Build history of the part. All positions in model axes, mm. Face numbers are marked on the shaded views. Coordinates: 2 decimals unless noted, no trailing zeros. Loops run counter-clockwise (first coordinate to the right, second up) from the corner with the lowest first, then second, coordinate; pieces in that order, holes last.
(1) Slice it at C-C (z = 15). Give the cut face in (x, y).
(2) Slice it at D-D (z = 11). Give the cut face in (x, y), and give its area (3 significant figures).
(3) Slice it at A-A (x = 0). Give the cut face in (y, z), and give its area (3 significant figures).
(4) Flat gauge pins, fed straight in: P1, Ø11, axis at x = 0, y = -14.82, coming from the +Z side; P2, Ø1, axis at y = -45.5, z = 16, coming from the -X side; P3, Ø5, axis at y = -46.5, z = -7, coming from the +X side. Where does each tip first touch, or does it go through?
(5) Wall check: L1, parallel to Y at x = 0, z = 14.25; L2, parallel to Y at x = -5.5, z = 10.5; L3, parallel to X at y = -37, z = 17. Give the ranges that are in metal, low to high.
(6) Two-plate mould, pull along Y, no slides. Class the marked faces 1, 2 and 3: pulls with the +Y half, pulls with the -Y half, needs draft (parallel to the pull), parting line crosses it, or undercut.
(7) Slice it at B-B (y = -44). Give the cut face in (x, z), and give its area (3 significant figures).
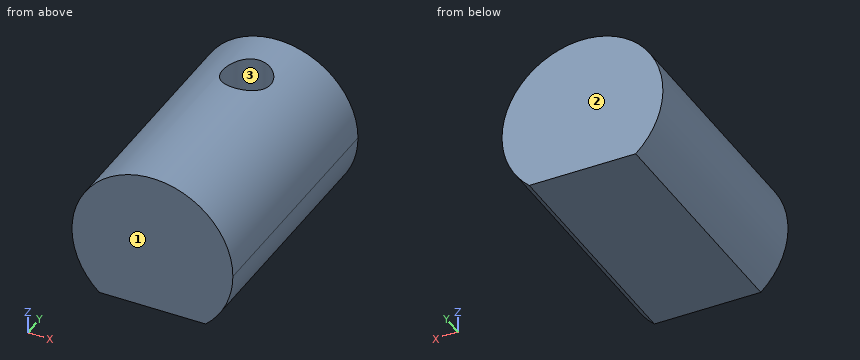
from build123d import *

# Parameters (mm, degrees)
F0_R     = 20
F1_DEPTH = 60
F3_R     = 6
F4_DEPTH = 23.59607
F5_W     = 79.34783
F5_H     = 17.173914
F6_DEPTH = 121.24079


with BuildPart() as f1:
    # F0 (on Front) → F1 (new body)
    with BuildSketch(Plane.XZ):
        Circle(F0_R)
    extrude(amount=F1_DEPTH)

    # F3 (on offset) → F4 (cut)
    with BuildSketch(Plane.XY.offset(10)):
        with Locations((0, -14.817017)):
            Circle(F3_R)
    extrude(amount=F4_DEPTH, mode=Mode.SUBTRACT)

    # F5 (on face) → F6 (cut)
    with BuildSketch(Plane.XZ.offset(60)):
        with Locations((7.579689, -23.586957)):
            Rectangle(F5_W, F5_H)
    extrude(amount=-F6_DEPTH, mode=Mode.SUBTRACT)


solid = f1.part
Response values:
1. outline: (-13.23, -60) - (13.23, -60) - (13.23, 0) - (-13.23, 0) - close; hole circle Ø12 at (0, -14.82)
2. outline: (-16.7, -60) - (16.7, -60) - (16.7, 0) - (-16.7, 0) - close; hole circle Ø12 at (0, -14.82)
2. area: 1,890 mm2
3. outline: (-60, -15) - (0, -15) - (0, 20) - (-8.82, 20) - (-8.82, 10) - (-20.82, 10) - (-20.82, 20) - (-60, 20) - close
3. area: 1,980 mm2
4. P1: stops at z = 10
4. P2: stops at x = -12.64
4. P3: stops at x = 19.49
5. L1: y = -60 to -20.82, -8.82 to 0
5. L2: y = -60 to -17.21, -12.42 to 0
5. L3: x = -10.54 to 10.54
6. face 1: pulls with the -Y half
6. face 2: pulls with the +Y half
6. face 3: undercut
7. outline: (-13.23, -15) - (13.23, -15) arc R20 ccw (long way) to start
7. area: 1,170 mm2
